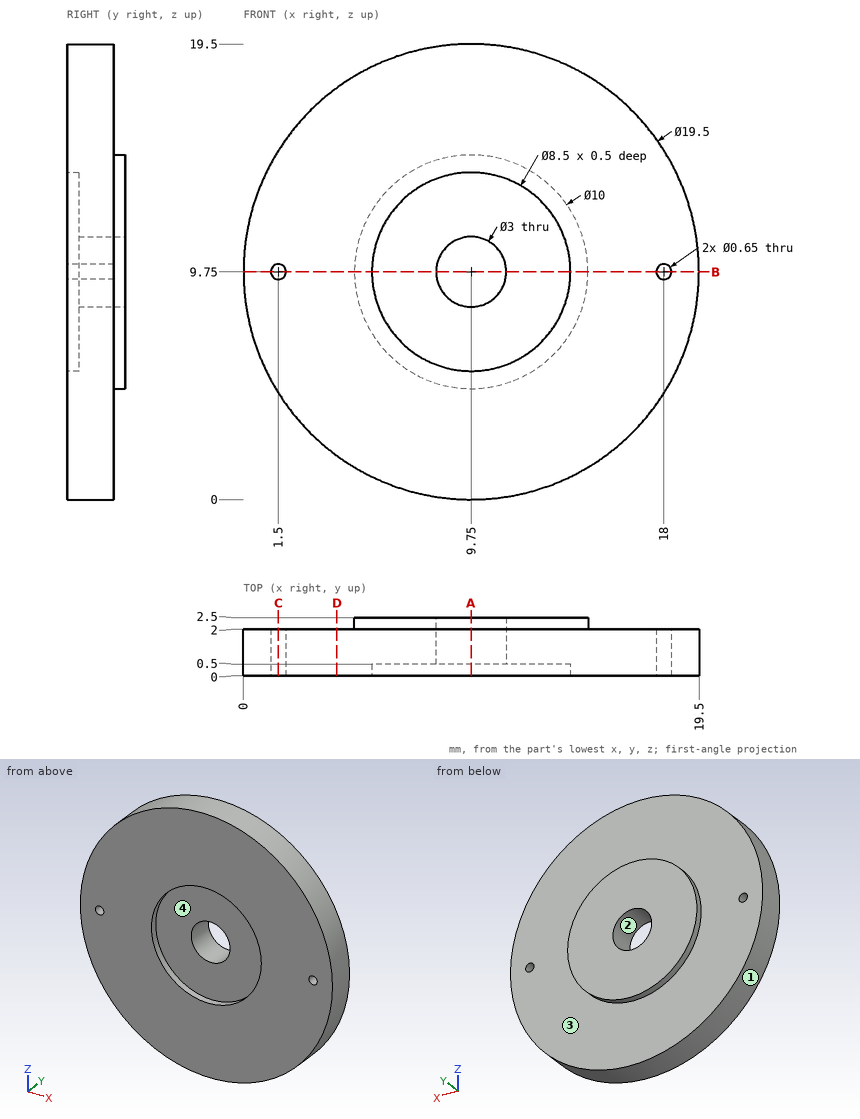
The drawing under review shows one solid part. Ordinate dimensions are in mm from its lowest x, y, z. Coordinates: 2 decimals unless noted, no trailing zeros. Loops run counter-clockwise (first coordinate to the right, second up) from the corner with the lowest first, then second, coordinate; pieces in that order, holes last. Notation, with made-up numbers: M -8.5,35 L 33.5,35 A16 ccw 33.5,42 Z; hole C 39,56 d6. An arc over 180 degrees is marked long. Use one line per item in the form item = value.
(1) Consider section A-A (x = 9.75). Write out the cut boundary in (y, z).
Return value:
outline = M 0,0 L 2,0 L 2,4.75 L 2.5,4.75 L 2.5,8.25 L 0.5,8.25 L 0.5,5.5 L 0,5.5 Z; M 0,14 L 0.5,14 L 0.5,11.25 L 2.5,11.25 L 2.5,14.75 L 2,14.75 L 2,19.5 L 0,19.5 Z
(2) For line 1 along Z through (x, y) = (9.75, 1.3); line 2 along Z through (x, y) = (9.75, 0.35); line 3 along Y through (x, z) = (13.75, 14.5), list the stretches that pass through material, from the lowest coordinate up. Write a range as from..to.
Return value:
line_1 = 0..8.25, 11.25..19.5
line_2 = 0..5.5, 14..19.5
line_3 = 0..2
(3) Consider section D-D (x = 4). Write out the cut boundary in (y, z), and give its area (3 significant figures).
Return value:
outline = M 0,1.88 L 2,1.88 L 2,17.62 L 0,17.62 Z
area = 31.5 mm2
(4) Consider section B-B (z = 9.75). Write out the cut boundary in (x, y) (3 decimals), and give its area (4 significant figures).
Return value:
outline = M 0,0 L 1.175,0 L 1.175,2 L 0,2 Z; M 1.825,0 L 5.5,0 L 5.5,0.5 L 8.25,0.5 L 8.25,2.5 L 4.75,2.5 L 4.75,2 L 1.825,2 Z; M 11.25,0.5 L 14,0.5 L 14,0 L 17.675,0 L 17.675,2 L 14.75,2 L 14.75,2.5 L 11.25,2.5 Z; M 18.325,0 L 19.5,0 L 19.5,2 L 18.325,2 Z
area = 31.15 mm2
(5) Draft analysis for pull direction X (two halves, no side actions). For the marked faces 1, 2, 3 and 4, state which applies: pulls with the +X half, pulls with the -X half, needs draft (parallel to the pull), parting line crosses it, or undercut.
Return value:
face_1 = parting line crosses it
face_2 = undercut
face_3 = needs draft
face_4 = undercut
(6) Clearance check with flat-ended pins moving along their axes: P1, Ø1, axis at x = 15.5, z = 15, coming from the +Y side; P2, Ø2.5, axis at x = 9.75, z = 9.75, coming from the +Y side. State where each tip first meets the part, or that it passes through.
Return value:
P1 = 2
P2 = through
(7) Consider section C-C (x = 1.5). Write out the cut boundary in (y, z) (3 decimals).
Return value:
outline = M 0,4.554 L 2,4.554 L 2,9.425 L 0,9.425 Z; M 0,10.075 L 2,10.075 L 2,14.946 L 0,14.946 Z
